Geometry: see drawing. Coordinates: mm, zero at the bounding-box minimum. Coordinates: 2 decimals unless noted, no trailing zeros. Order: outer loops, then holes, each group sorted by start corner. A loop starts at its lowest first (then second) coordinate and runs counter-clockwise, first axis right, second up.
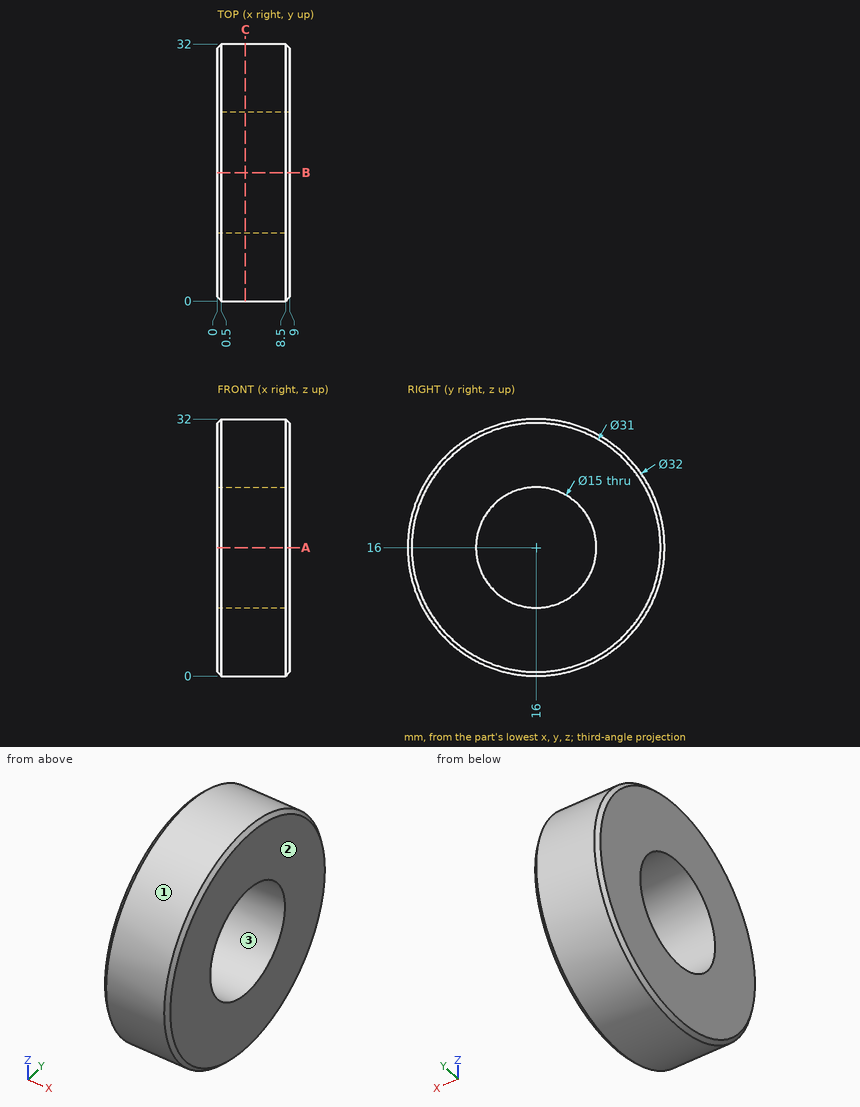
Q1. Section query A-A on z = 16. Output: boundary loops of the cut face in (x, y).
Solutions:
outline: (0, 0.5) - (0.5, 0) - (8.5, 0) - (9, 0.5) - (9, 8.5) - (0, 8.5) - close; (0, 23.5) - (9, 23.5) - (9, 31.5) - (8.5, 32) - (0.5, 32) - (0, 31.5) - close
Q2. Pull-direction query (Z, two-part tool) for the marked faces 1, 2 and 3; classes: pulls with the +Z half, pulls with the -Z half, needs draft (parallel to the pull), parting line crosses it, or undercut.
Solutions:
face 1: parting line crosses it
face 2: needs draft
face 3: undercut
Q3. Material intervals for line 1 along Z through (x, y) = (2.25, 16); line 2 along Y through (x, z) = (8.5, 15); line 3 along Z through (x, y) = (7.25, 10), sorted ascending.
Solutions:
line 1: z = 0 to 8.5, 23.5 to 32
line 2: y = 0.03 to 8.57, 23.43 to 31.97
line 3: z = 1.17 to 11.5, 20.5 to 30.83
Q4. Section query C-C on x = 3.5. Output: boundary loops of the cut face in (y, z).
Solutions:
outline: circle Ø32 at (16, 16); hole circle Ø15 at (16, 16)
Q5. Pin query (flat end, axial travel): P1, Ø1, axis at x = 5, z = 28, coming from the -Y side; P2, Ø1.5, axis at x = 7, y = 13.5, coming from the +Z side; P3, Ø3, axis at x = 3.5, z = 24, coming from the -Y side. Return the tip coordinate at first contact, or that it passes through.
Solutions:
P1: stops at y = 4.88
P2: stops at z = 31.9
P3: stops at y = 1.38
